Can you work these out from the drawing? Everything is in mm from the part's minimum corner. Coordinates: 2 decimals unless noted, no trailing zeros. Write each loop counter-clockwise with the first axis right and the second up, starting at its lowest first coordinate (ties: lowest second). Pieces come first, ordered by that corner, then holes.
(1) For pin 1 Ø10 at (x, z) = (29, 132.5) entering from +Y, with a flat end and sliding along its axis, tell me the tip position at first contact or that it passes through.
(2) Please list where these lines run through material, in increasing order: probe 1 along Z at (x, y) = (106.5, 2.3); probe 2 along X at (y, z) = (0.3, 26).
(3) Imagine slicing it at C-C, the plane y = 1.6. List the corners of the cut face in (x, z) for me, plus the area to 3 significant figures.
(4) Imagine slicing it at A-A, the plane x = 115. List the corners of the cut face in (y, z) for me.
(5) Imagine slicing it at B-B, the plane z = 65. List the corners of the cut face in (x, y) for me, plus the area to 3 significant figures.
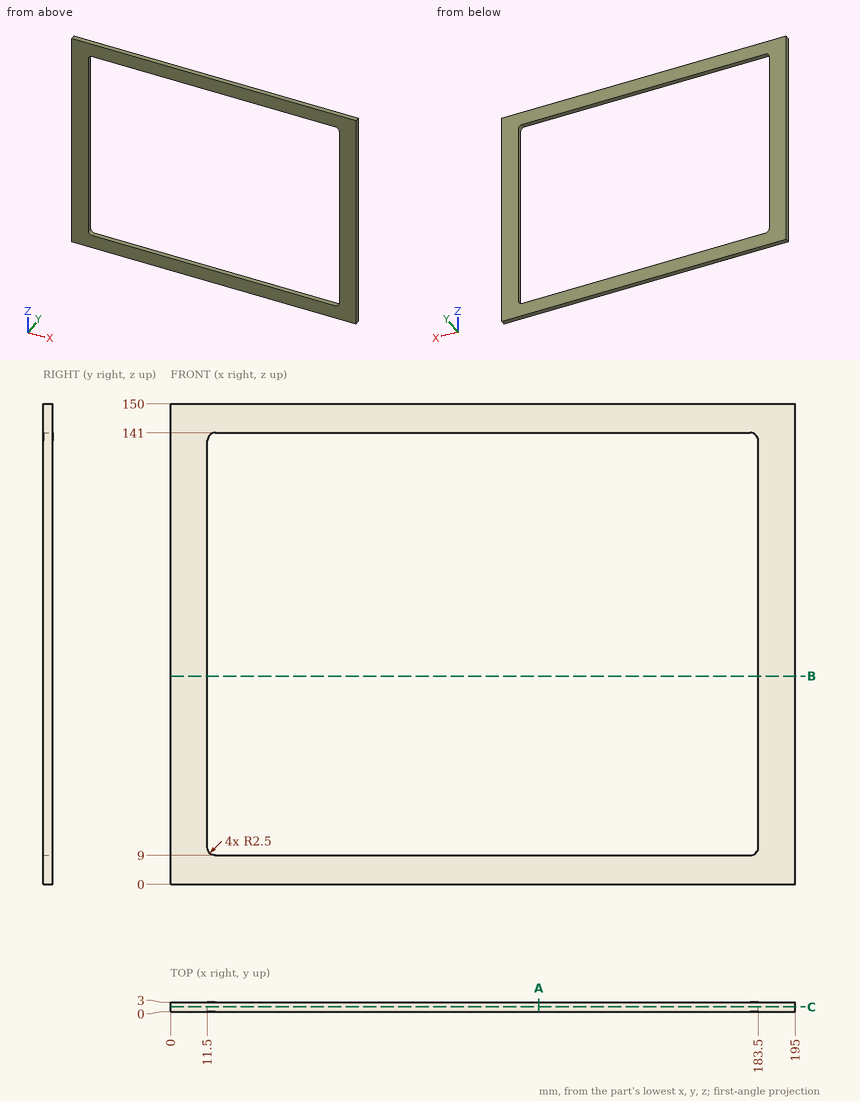
Recorded:
1. pin 1: passes through
2. probe 1: z = 0 to 9, 141 to 150
2. probe 2: x = 0 to 11.5, 183.5 to 195
3. outline: (0, 0) - (195, 0) - (195, 150) - (0, 150) - close; hole (11.5, 11.5) arc R2.5 ccw to (14, 9) - (181, 9) arc R2.5 ccw to (183.5, 11.5) - (183.5, 138.5) arc R2.5 ccw to (181, 141) - (14, 141) arc R2.5 ccw to (11.5, 138.5) - close
3. area: 6,550 mm2
4. outline: (0, 0) - (3, 0) - (3, 9) - (0, 9) - close; (0, 141) - (3, 141) - (3, 150) - (0, 150) - close
5. outline: (0, 0) - (11.5, 0) - (11.5, 3) - (0, 3) - close; (183.5, 0) - (195, 0) - (195, 3) - (183.5, 3) - close
5. area: 69.0 mm2
